Check sheet for the modelled part. Datum: model origin and axes. Units: mm. Face numbers are marked on the shaded views. A direction names the side the tool comes from. Round coordinates to 2 decimals unless told otherwise and drop trailing zeros. Order: outer loops, then holes, each group sorted by start corner. A loop starts at its lowest first (then second) coordinate and runs counter-clockwise, first axis right, second up. Notation, with made-up numbers: M 79.25,25 L 121.25,25 A30 cw 121.25,53 Z; hole C 31.25,-2 d5. An arc over 180 degrees is marked long. One line per item, written item: value. Start each with the question number.
(1) Release check for a two-part mould opening along X. For the marked faces 4, 5 and 6 record: released by +X, released by -X, zero draft, split by the parting line, or undercut.
(2) Depth check by flat-ended pin: pin 1 Ø2 at (x, z) = (-2, 0) entering from -Y; pin 2 Ø0.5 at (x, y) = (-0.5, 0.5) entering from +Z; pin 3 Ø4 at (x, y) = (-3, 7) entering from +Z; pin 4 Ø0.8 at (x, y) = (1, 0.5) entering from -Z. Enter the tip coordinate at first touch or a pass-through.
(3) Cross-section at B-B, the plane x = 0. Enter the section's corners in (y, z) (3 decimals), and give its area (3 significant figures).
(4) Cross-section at C-C, the plane x = 1.5. Enter the section's corners in (y, z), and give its area (3 significant figures).
(5) Access from +Z, -Z, +X, -X, +Y, -Y to the whole of each face (thin tool, end or side, straight path). Record for the marked faces 1, 2 and 3.
(6) Thickness scan on L1, parallel to X at y = 9.75, z = -0.2; L2, parallel to X at y = 9, z = 0.65; L3, parallel to Y at x = -1, z = -1.85. Record the ranges inside material, lowest first.
(7) Cross-section at A-A, the plane y = 10.25. Enter the section's corners in (x, z) (3 decimals).
Autodesk Inventor part; units mm, degrees
ref_plane "YZ Plane" through (0, 0, 0) normal (1, 0, 0) x (0, 1, 0)
ref_plane "XZ Plane" through (0, 0, 0) normal (0, 1, 0) x (-1, 0, 0)
ref_plane "XY Plane" through (0, 0, 0) normal (0, 0, 1) x (1, 0, 0)
sketch "Sketch1" plane through (0, 0, 0) normal (0, 1, 0) x (-1, 0, 0)
  line L0 (-2.5, -1.75) -> (2.5, -1.75)
  line L1 (2.5, -1.75) -> (2.5, 1.75)
  line L2 (2.5, 1.75) -> (-2.5, 1.75)
  line L3 (-2.5, 1.75) -> (-2.5, -1.75)
  line L4 (-2.5, -1.75) -> (2.5, 1.75) construction
  line L5 (2.5, -1.75) -> (-2.5, 1.75) construction
  point P0 (0, 0)
  dimension "d0" = 5
  dimension "d1" = 3.5
extrude "Extrusion1" add sketch "Sketch1" along normal blind 1
sketch "Sketch2" plane through (0, 1, 0) normal (0, 1, 0) x (1, 0, 0)
  line L0 (-3.9, -2.25) -> (3.9, -2.25)
  line L1 (3.9, -2.25) -> (3.9, 2.25)
  line L2 (3.9, 2.25) -> (-3.9, 2.25)
  line L3 (-3.9, 2.25) -> (-3.9, -2.25)
  line L4 (-3.9, -2.25) -> (3.9, 2.25) construction
  line L5 (3.9, -2.25) -> (-3.9, 2.25) construction
  point P0 (0, 0)
  dimension "d4" = 7.8
  dimension "d5" = 4.5
extrude "Extrusion2" add sketch "Sketch2" along normal blind 1
sketch "Sketch3" plane through (0, 2, 0) normal (0, 1, 0) x (1, 0, 0)
  line L0 (-2.75, -1.5) -> (2.75, -1.5)
  line L1 (2.75, -1.5) -> (2.75, 1.5)
  line L2 (2.75, 1.5) -> (-2.75, 1.5)
  line L3 (-2.75, 1.5) -> (-2.75, -1.5)
  line L4 (-2.75, -1.5) -> (2.75, 1.5) construction
  line L5 (2.75, -1.5) -> (-2.75, 1.5) construction
  point P0 (0, 0)
  dimension "d8" = 5.5
  dimension "d9" = 3
extrude "Extrusion3" add sketch "Sketch3" along normal blind 4.5 draft -6
fillet "Fillet1" radius 0.3 8 edges at (2.5135, 4.25, 1.2635) (-2.5135, 4.25, 1.2635) (0, 2, 1.5) (2.75, 2, 0) (2.5135, 4.25, -1.2635) (0, 2, -1.5) (-2.5135, 4.25, -1.2635) (-2.75, 2, 0)
fillet "Fillet2" radius 0.15 20 edges at (0, 2, 2.25) (3.9, 2, 0) (0, 2, -2.25) (-3.9, 2, 0) (-3.9, 1, 0) (-3.9, 1.5, 2.25) (-3.9, 1.5, -2.25) (0, 1, -2.25) (3.9, 1.5, -2.25) (0, 1, 2.25) (3.9, 1.5, 2.25) (3.9, 1, 0) (-2.1898, 6.5, -0.9398) (-2.277, 6.5, 0) (-2.1898, 6.5, 0.9398) (0, 6.5, 1.027) (2.1898, 6.5, 0.9398) (2.277, 6.5, 0) (2.1898, 6.5, -0.9398) (0, 6.5, -1.027)
sketch "Sketch4" plane through (0, 6.5, 0) normal (0, 1, 0) x (1, 0, 0)
  circle A0 centre (0, 0) radius 0.72
  circle A1 centre (1.44, 0) radius 0.72
  circle A2 centre (-1.44, 0) radius 0.72
  dimension "d14" = 1.44
  dimension "d15" = 1.44
  dimension "d16" = 1.44
extrude "Extrusion4" add sketch "Sketch4" along normal blind 3
sketch "Sketch5" plane through (-1.44, 9.5, 0) normal (0, 1, 0) x (1, 0, 0)
  circle A0 centre (0, 0) radius 0.72
  arc A1 (0.72, 0) -> (2.16, 0) centre (1.44, 0) ccw
  arc A2 (2.16, 0) -> (0.72, 0) centre (1.44, 0) ccw
  circle A3 centre (2.88, 0) radius 0.72
  circle A4 centre (0, 0) radius 0.375
  circle A5 centre (1.44, 0) radius 0.375
  circle A6 centre (2.88, 0) radius 0.375
  dimension "d20" = 0.75
  dimension "d21" = 0.75
extrude "Extrusion5" add sketch "Sketch5" along normal blind 1 contours A4 | A5 | A6
properties part number "wire" material "PET Plastic"
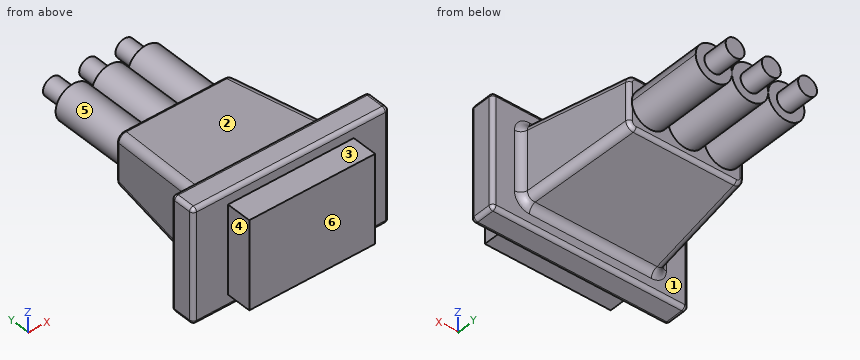
Values found:
1. face 4: released by -X
1. face 5: undercut
1. face 6: zero draft
2. pin 1: y = 0
2. pin 2: z = 1.75
2. pin 3: z = 1.16
2. pin 4: z = -1.75
3. outline: M 0,-1.75 L 1,-1.75 L 1,-2.1 A0.15 ccw 1.15,-2.25 L 1.85,-2.25 A0.15 ccw 2,-2.1 L 2,-1.77 A0.3 cw 2.269,-1.472 L 6.366,-1.041 A0.15 ccw 6.5,-0.892 L 6.5,-0.72 L 9.5,-0.72 L 9.5,-0.375 L 10.5,-0.375 L 10.5,0.375 L 9.5,0.375 L 9.5,0.72 L 6.5,0.72 L 6.5,0.892 A0.15 ccw 6.366,1.041 L 2.269,1.472 A0.3 cw 2,1.77 L 2,2.1 A0.15 ccw 1.85,2.25 L 1.15,2.25 A0.15 ccw 1,2.1 L 1,1.75 L 0,1.75 Z
3. area: 24.4 mm^2
4. outline: M 0,-1.75 L 1,-1.75 L 1,-2.1 A0.15 ccw 1.15,-2.25 L 1.85,-2.25 A0.15 ccw 2,-2.1 L 2,-1.77 A0.3 cw 2.27,-1.47 L 6.37,-1.04 A0.15 ccw 6.5,-0.89 L 6.5,-0.72 L 9.5,-0.72 L 9.5,-0.37 L 10.5,-0.37 L 10.5,0.37 L 9.5,0.37 L 9.5,0.72 L 6.5,0.72 L 6.5,0.89 A0.15 ccw 6.37,1.04 L 2.27,1.47 A0.3 cw 2,1.77 L 2,2.1 A0.15 ccw 1.85,2.25 L 1.15,2.25 A0.15 ccw 1,2.1 L 1,1.75 L 0,1.75 Z
4. area: 24.4 mm^2
5. face 1: +Y
5. face 2: +Z, +X, -X, +Y
5. face 3: +Z, +X, -X, -Y
6. L1: -1.76 to -1.12, -0.32 to 0.32, 1.12 to 1.76
6. L2: -1.75 to -1.13, -0.31 to 0.31, 1.13 to 1.75
6. L3: 1 to 2
7. outline: C -1.44,0 d0.75; C 0,0 d0.75; C 1.44,0 d0.75
